Design review of the part built by this model. Coordinates are the model's own, in mm. A direction names the side the tool comes from. Coordinates: 2 decimals unless noted, no trailing zeros. Write each loop counter-clockwise with the first axis right and the second up, starting at its lowest first coordinate (ties: lowest second). Pieces come first, ordered by that corner, then holes. Notation, with made-up numbers: M 47.25,49.5 L 104.25,49.5 A23 cw 104.25,59.5 Z; hole C -11,70 d4. An arc over 180 degrees is marked long. Write item = value, one per line.
Autodesk Inventor part; units mm, degrees
ref_plane "Work Plane1" through (0, 0, 16) normal (0, 0, 1) x (1, 0, 0)
ref_plane "YZ Plane" through (0, 0, 0) normal (1, 0, 0) x (0, 1, 0)
ref_plane "XZ Plane" through (0, 0, 0) normal (0, 1, 0) x (-1, 0, 0)
sketch "Sketch1" plane through (0, 0, 0) normal (0, 0, 1) x (1, 0, 0)
  arc A0 (0, 22) -> (-22, 0) centre (0, 0) ccw
  arc A1 (0, 17.25) -> (-17.25, 0) centre (38.3744, -38.3744) ccw
  line L0 (0, 17.25) -> (0, 22)
  line L1 (-17.25, 0) -> (-22, 0)
  dimension "d0" = 44
ref_plane "Work Plane1" through (0, 0, 16) normal (0, 0, 1) x (1, 0, 0)
extrude "Extrusion3" add sketch "Sketch1" along normal blind 11
sketch "Sketch5" plane through (0, 0, 11) normal (0, 0, 1) x (1, 0, 0)
  arc A0 (0, 17.25) -> (-17.25, 0) centre (38.3744, -38.3744) ccw
  line L0 (-4.3084, 0) -> (-17.25, 0)
  line L1 (-2.75, 0) -> (-17.25, 0)
  circle A1 centre (0, 0) radius 1.525
  arc A2 (-2.4943, -1.1579) -> (1.1579, 2.4943) centre (0, 0) ccw
  line L2 (0, 17.25) -> (0, 4.3084)
  line L3 (-17.25, 0) -> (-2.75, 0)
  arc A3 (0, 4.3084) -> (1.1579, 2.4943) centre (2, 4.3084) ccw
  arc A4 (-2.4943, -1.1579) -> (-4.3084, 0) centre (-4.3084, -2) ccw
  point P0 (0, 2.75)
  dimension "d25" = 3.05
  dimension "d26" = 5.5
  dimension "d27" = 2
extrude "Extrusion4" add sketch "Sketch5" against normal blind 3
sketch "Sketch6" plane through (0, 0, 0) normal (0, 0, -1) x (-1, 0, 0)
  line L0 (0, 0) -> (15.5563, 15.5563)
  arc A0 (22, 0) -> (0, 22) centre (0, 0) ccw
  line L1 (0, 0) -> (22, 0) construction
  circle A1 centre (12.1976, 12.1976) radius 2.8
  dimension "d30" = 45
  dimension "d31" = 5.6
  dimension "d32" = 17.25
extrude "Extrusion5" cut sketch "Sketch6" against normal blind 3
properties part number "led-holder"
Q1. The part is to be moulded in two halves that separate along X. For faces 1 (the cylindrical face through (-11.591, 9.464, 1.479)), 2 (the cylindrical face through (-1.524, 0.067, 9.521)), 3 (the cylindrical face through (0.306, 3.246, 9.521)), 4 (the flat face through (-5, 5, 8)), say which applies: +X half, -X half, draft (parallel to the pull), parting line (faces both ways), or undercut.
Check result:
face_1 = undercut
face_2 = undercut
face_3 = +X half
face_4 = draft
Q2. Wall thickness on line 1 (Z direction, x = 0, y = 2); line 2 (X direction, y = 14, z = 1); line 3 (X direction, y = 9.75, z = 2.5): over which ranges is each line inside the solid? List them lowest first.
Check result:
line_1 = 8 to 11
line_2 = -16.97 to -14.34, -10.05 to -4.33
line_3 = -19.72 to -13.56, -10.84 to -9.07
Q3. Consider section D-D, the plane z = 2. State the section outline as (x, y) points.
Check result:
outline = M -22,0 L -17.25,0 A67.58 cw 0,17.25 L 0,22 A22 ccw Z; hole C -12.2,12.2 d5.6
Q4. Machinability: for faces 5 (the flat face through (-9, 11, 0)), 6 (the flat face through (0, 17, 9)), 7 (the cylindrical face through (-9.53, 9.29, 3.94)), 8 (the flat face through (-17, 0, 9)), 9 (the flat face through (-12, 12, 3)), which of the approach directions +Z, -Z, +X, -X, +Y, -Y give a long, thin tool a straight path to every point of the face, cutting with its end or side? Answer none if there is none.
Check result:
face_5 = -Z, +X, -X, +Y, -Y
face_6 = +Z, -Z, +X, +Y
face_7 = -Z, +X, -Y
face_8 = +Z, -Z, -X, -Y
face_9 = -Z
Q5. Consider section A-A, the plane y = 13.5. State the section outline as (x, z) points, and give its area (3 significant figures).
Check result:
outline = M -17.37,0 L -14.68,0 L -14.68,3 L -9.72,3 L -9.72,0 L -4.94,0 L -4.94,8 L 0,8 L 0,11 L -17.37,11 Z
area = 137 mm²
Q6. For P1, Ø3, axis at x = -17, z = 6, coming from the +Y side; P2, Ø3.5, axis at y = 14, z = 7.5, coming from the +X side; P3, Ø6.5, axis at x = -12.2, y = 12.2, coming from the -Z side; P4, Ø1, axis at x = -17.5, z = 7.5, coming from the -Y side, all flat-tipped, find the tip position at first contact; note any pin that passes through.
Check result:
P1 = 15.61
P2 = 0
P3 = 0
P4 = 0
Q7. Consider section C-C, the plane z = 7.25. State the section outline as (x, y) points.
Check result:
outline = M -22,0 L -17.25,0 A67.58 cw 0,17.25 L 0,22 A22 ccw Z
Q8. Consider section B-B, the plane x = -10.25. State the section outline as (y, z) points, and give its area (3 significant figures).
Check result:
outline = M 0,8 L 8.55,8 L 8.55,0 L 10.19,0 L 10.19,3 L 14.21,3 L 14.21,0 L 19.47,0 L 19.47,11 L 0,11 Z
area = 134 mm²
